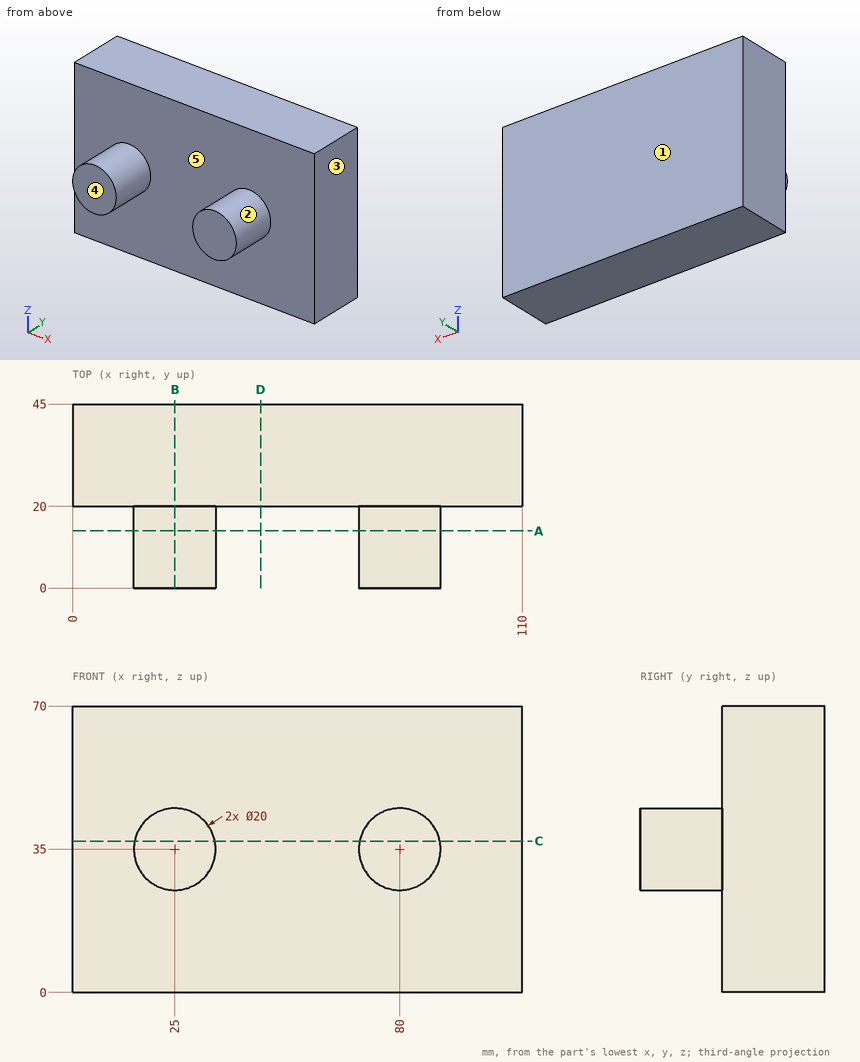
Source: three-view drawing plus pictorial views. Frame: mm from the lowest corner of the part. A direction names the side the tool comes from. Round coordinates to 2 decimals unless told otherwise and drop trailing zeros. Order: outer loops, then holes, each group sorted by start corner. A loop starts at its lowest first (then second) coordinate and runs counter-clockwise, first axis right, second up. Notation, with made-up numbers: (-35, -16.5) - (-13, -16.5) arc R14 ccw to (-13, 5.5) - close; hole circle Ø9 at (-0.75, 69). An arc over 180 degrees is marked (long way). Use a Markdown table: item, result.
1. First-contact query: pin 1 (12 mm diameter, centred on x = 43, z = 29, fed in from -Y); pin 2 (2 mm diameter, centred on y = 9, z = 29.5, fed in from -X); pin 3 (8 mm diameter, centred on y = 10.5, z = 38.5, fed in from -X). Flat tips, straight axial feed; report the tip coordinate or a pass-through.
Evaluation:
| item | result |
|---|---|
| pin 1 | y = 20 |
| pin 2 | x = 16.07 |
| pin 3 | x = 15 |
2. Section A-A on y = 14. Return the cut outline in (x, z).
Evaluation:
| item | result |
|---|---|
| outline | circle Ø20 at (25, 35); circle Ø20 at (80, 35) |
3. Section C-C on z = 37. Return the cut outline in (x, y), then the cut area to 3 significant figures.
Evaluation:
| item | result |
|---|---|
| outline | (0, 20) - (15.2, 20) - (15.2, 0) - (34.8, 0) - (34.8, 20) - (70.2, 20) - (70.2, 0) - (89.8, 0) - (89.8, 20) - (110, 20) - (110, 45) - (0, 45) - close |
| area | 3,530 mm^2 |
4. Material intervals for probe 1 along Y at (x, z) = (29.5, 12); probe 2 along Z at (x, y) = (80, 14.5); probe 3 along X at (y, z) = (17, 43.5), sorted ascending.
Evaluation:
| item | result |
|---|---|
| probe 1 | 20 to 45 |
| probe 2 | 25 to 45 |
| probe 3 | 19.73 to 30.27, 74.73 to 85.27 |
5. Access query for the marked faces 4 and 5. Directions: +Z, -Z, +X, -X, +Y, -Y. A direction counts if a zero-diameter tool reaches every point of the face in a straight line with its end or side. Return the directions, or none.
Evaluation:
| item | result |
|---|---|
| face 4 | +Z, -Z, +X, -X, -Y |
| face 5 | -Y |
6. Section D-D on x = 46. Return the cut outline in (y, z), then the cut area to 3 significant figures.
Evaluation:
| item | result |
|---|---|
| outline | (20, 0) - (45, 0) - (45, 70) - (20, 70) - close |
| area | 1,750 mm^2 |
7. Section B-B on x = 25. Return the cut outline in (y, z).
Evaluation:
| item | result |
|---|---|
| outline | (0, 25) - (20, 25) - (20, 0) - (45, 0) - (45, 70) - (20, 70) - (20, 45) - (0, 45) - close |
8. Mould query, pull axis X, two halves, no side actions, for the marked faces 1, 2 and 3. Classes: +X half, -X half, draft (parallel to the pull), parting line (faces both ways), or undercut.
Evaluation:
| item | result |
|---|---|
| face 1 | draft |
| face 2 | undercut |
| face 3 | +X half |
